Verification items for the finished model (mm, model axes). Face numbers are marked on the shaded views. Coordinates: 2 decimals unless noted, no trailing zeros. Order: outer loops, then holes, each group sorted by start corner. A loop starts at its lowest first (then second) coordinate and runs counter-clockwise, first axis right, second up. Notation, with made-up numbers: M 12,-28 L 25,-28 A17 cw 25,-11 Z; hole C 86.5,48.5 d7. An arc over 180 degrees is marked long. Return JSON: item names as keys, results as strings.
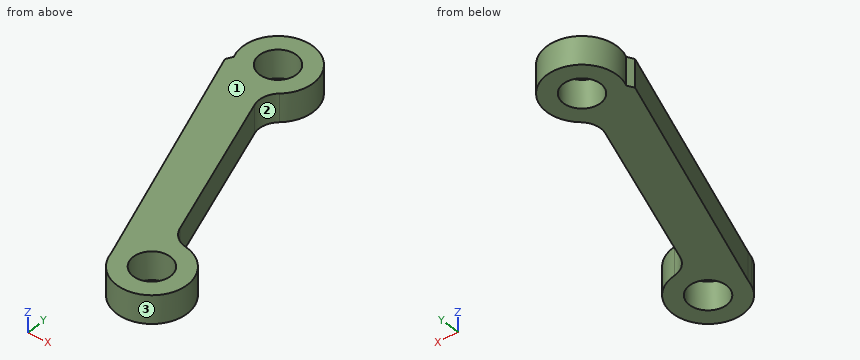
```python
from build123d import *

# Parameters (mm, degrees)
SKETCH1_R           = 2.6375
BOSS_EXTRUDE1_DEPTH = 4


with BuildPart() as part:
    # Sketch1 → Boss-Extrude1 (new body)
    with BuildSketch(Plane.XY.offset(4)):
        with BuildLine():
            Line((18.121313038, 57.499552699), (11.130625568, 79.363045761))
            ThreePointArc((11.130625568, 79.363045761), (11.103854309, 81.101969158), (12.046376558, 82.563551551))
            ThreePointArc((12.046376558, 82.563551551), (9.982846794, 91.235495297), (4.191986809, 84.458570917))
            Line((4.191986809, 84.458570917), (3.669492538, 83.571702076))
            Line((3.669492538, 83.571702076), (14.841853522, 49.779462629))
            Line((14.841853522, 49.779462629), (15.118467898, 48.820925017))
            ThreePointArc((15.118467898, 48.820925017), (23.681425942, 47.199148201), (20.62266155, 55.359930695))
            ThreePointArc((20.62266155, 55.359930695), (19.067995929, 56.074357266), (18.121313038, 57.499552699))
        make_face()
        with Locations(Location((19.856196321, 50.419026825, 0), (0, 0, 180))):
            Circle(SKETCH1_R, mode=Mode.SUBTRACT)
        with Locations(Location((8.810151598, 86.374961789, 0), (0, 0, 180))):
            Circle(SKETCH1_R, mode=Mode.SUBTRACT)
    extrude(amount=-BOSS_EXTRUDE1_DEPTH)


solid = part.part
```
Q1. Cross-section at D-D, the plane y = 68.5. Record the boundary of the cut face in (x, z), and give its area (3 significant figures).
Values:
{"outline": "M 8.65,0 L 14.6,0 L 14.6,4 L 8.65,4 Z", "area": "23.8 mm^2"}
Q2. Cross-section at C-C, the plane x = 22. Record the boundary of the cut face in (y, z), and give its area (3 significant figures).
Values:
{"outline": "M 45.9,0 L 48.88,0 L 48.88,4 L 45.9,4 Z; M 51.96,0 L 54.94,0 L 54.94,4 L 51.96,4 Z", "area": "23.8 mm^2"}
Q3. Draft check along Y on the marked faces 1, 2 and 3. Enter one of: pulls with the +Y half, pulls with the -Y half, needs draft (parallel to the pull), parting line crosses it, or undercut.
Values:
{"face 1": "needs draft", "face 2": "undercut", "face 3": "parting line crosses it"}
Q4. Go/stop test with a flat-tipped pin: pin 1 (1 mm diameter, centred on y = 55, z = 3.5, fed in from +X). Record where the tip stops, or that it passes through.
Values:
{"pin 1": "x = 22.75"}
Q5. Cross-section at A-A, the plane x = 13.25. Record the boundary of the cut face in (y, z), and give its area (3 significant figures).
Values:
{"outline": "M 54.59,0 L 72.73,0 L 72.73,4 L 54.59,4 Z; M 84.08,0 L 88.67,0 L 88.67,4 L 84.08,4 Z", "area": "91.0 mm^2"}
Q6. Cross-section at B-B, the plane z = 2.6. Record the boundary of the cut face in (x, y) (1 decimal).
Values:
{"outline": "M 3.7,83.6 L 14.8,49.8 L 15.1,48.8 A5 ccw long 20.6,55.4 A3.1 cw 18.1,57.5 L 11.1,79.4 A3 cw 12,82.6 A5 ccw long 4.2,84.5 Z; hole C 8.8,86.4 d5.3; hole C 19.9,50.4 d5.3"}
Q7. Material ranges on line 1 along Y through (x, z) = (19.25, 1.05); line 2 along Y through (x, z) = (21.5, 3.4); line 3 along X through (y, z) = (52.5, 0.4), recorded low to high.
Values:
{"line 1": "45.46 to 47.85, 52.99 to 55.93", "line 2": "45.7 to 48.36, 52.48 to 55.14", "line 3": "13.94 to 18.24, 21.48 to 24.4"}
